```python
from build123d import *

# Parameters (mm, degrees)
SKETCH_1_W          = 56.4
SKETCH_1_H          = 20
EXTRUDE_1_DEPTH     = 8
SKETCH_2_R          = 2.25
CUT_EXTRUDE_1_DEPTH = 8
CHAMFER_1_SIZE      = 3
SKETCH_3_R          = 20
CUT_EXTRUDE_2_DEPTH = 8
SKETCH_4_W          = 5
SKETCH_4_H          = 8
CUT_EXTRUDE_3_DEPTH = 8


with BuildPart() as part:
    # 스케치1 → 보스-돌출1 (new body)
    with BuildSketch(Plane(origin=(0, 0, 0), x_dir=(1, 0, 0), z_dir=(0, 1, 0))):
        with Locations((28.2, 10)):
            Rectangle(SKETCH_1_W, SKETCH_1_H)
    extrude(amount=EXTRUDE_1_DEPTH)

    # 스케치2 → 컷-돌출1 (cut)
    with BuildSketch(Plane(origin=(0, 8, 0), x_dir=(1, 0, 0), z_dir=(0, 1, 0))):
        with Locations(Location((51.75, 15.35, 0), (0, 0, 270))):
            Circle(SKETCH_2_R)
        with Locations(Location((4.65, 15.35, 0), (0, 0, 270))):
            Circle(SKETCH_2_R)
    extrude(amount=-CUT_EXTRUDE_1_DEPTH, mode=Mode.SUBTRACT)

    # 모따기1
    chamfer_1_edges = [part.edges().sort_by_distance(p)[0] for p in [
        (56.4, 4, 0),
        (0, 4, 0),
    ]]
    chamfer(chamfer_1_edges, length=CHAMFER_1_SIZE)

    # 스케치3 → 컷-돌출2 (cut)
    with BuildSketch(Plane(origin=(0, 8, 0), x_dir=(1, 0, 0), z_dir=(0, 1, 0))):
        with Locations((28.2, -8.2)):
            Circle(SKETCH_3_R)
    extrude(amount=-CUT_EXTRUDE_2_DEPTH, mode=Mode.SUBTRACT)

    # 스케치4 → 컷-돌출3 (cut)
    with BuildSketch(Plane(origin=(0, 8, 0), x_dir=(1, 0, 0), z_dir=(0, 1, 0))):
        with Locations((13.2, 16)):
            Rectangle(SKETCH_4_W, SKETCH_4_H)
        with Locations((43.2, 16)):
            Rectangle(SKETCH_4_W, SKETCH_4_H)
    extrude(amount=-CUT_EXTRUDE_3_DEPTH, mode=Mode.SUBTRACT)


solid = part.part
```
Model file for the job. Use its own axes, mm. A direction names the side the tool comes from. Coordinates: 2 decimals unless noted, no trailing zeros. Loops run counter-clockwise (first coordinate to the right, second up) from the corner with the lowest first, then second, coordinate; pieces in that order, holes last. Notation, with made-up numbers: M -5.75,-35.5 L 49.25,-35.5 A11 cw 49.25,-19.5 Z; hole C -2.75,61.5 d6. An arc over 180 degrees is marked long. Use CSV: the item, a comma, the result in double quotes. Start each with the question number.
1. Band-saw the part on D-D, the plane z = -4.5. List the corners of the cut face in (x, y).
2. Two-plate mould, pull along X, no slides. Class faces 3 (the flat face through (0, 4, -11)), 4 (the cylindrical face through (53.98, 4.06, -15.64)), 5 (the flat face through (15.7, 4, -16)), 6 (the flat face through (54.9, 3.9, -1.5)): pulls with the +X half, pulls with the -X half, needs draft (parallel to the pull), parting line crosses it, or undercut.
3. Probe probe 1 along X at (y, z) = (4, -15.35); probe 2 along X at (y, z) = (5, -12.5); probe 3 along X at (y, z) = (7.75, -8.25). List the from-to ranges inside material, lowest first. Write a range as [from, to].
4. Band-saw the part on A-A, the plane x = 51.75. List the corners of the cut face in (y, z), then the cut area to 3 significant figures.
5. Tool access for faces 1 (the flat face through (40.7, 4, -16)), 2 (the flat face through (6, 4, 0)): list every direction of +Z, -Z, +X, -X, +Y, -Y with a clear straight run to the whole face (end or side of a thin tool).
6. Band-saw the part on C-C, the plane y = 4.25. List the corners of the cut face in (x, z), then the cut area to 3 significant figures.
7. Flat gauge pins, fed straight in: pin 1 (1.5 mm diameter, centred on x = 29, y = 5.5, fed in from +Z); pin 2 (2 mm diameter, centred on x = 24.5, y = 2, fed in from +Z); pin 3 (1.5 mm diameter, centred on x = 13.5, y = 5.5, fed in from -Z); pin 4 (4 mm diameter, centred on x = 4.65, z = -15.35, fed in from +Y). Where does each tip first touch, or does it go through?
8. Band-saw the part on B-B, the plane z = -14. List the corners of the cut face in (x, y).
Entries:
1,outline,"M 0,0 L 12.75,0 L 12.75,8 L 0,8 Z; M 43.65,0 L 56.4,0 L 56.4,8 L 43.65,8 Z"
2,face 3,"pulls with the -X half"
2,face 4,"undercut"
2,face 5,"undercut"
2,face 6,"pulls with the +X half"
3,probe 1,"x = [0, 2.4], [6.9, 10.7], [15.7, 40.7], [45.7, 49.5], [54, 56.4]"
3,probe 2,"x = [0, 10.7], [15.7, 40.7], [45.7, 56.4]"
3,probe 3,"x = [0, 16.82], [39.58, 56.4]"
4,outline,"M 0,-20 L 8,-20 L 8,-17.6 L 0,-17.6 Z; M 0,-13.1 L 8,-13.1 L 8,0 L 0,0 Z"
4,area,"124 mm2"
5,face 1,"-Z, +Y, -Y"
5,face 2,"+Z, +X, -X, +Y, -Y"
6,outline,"M 0,-20 L 10.7,-20 L 10.7,-12 L 15.7,-12 L 15.7,-20 L 40.7,-20 L 40.7,-12 L 45.7,-12 L 45.7,-20 L 56.4,-20 L 56.4,-3 L 53.4,0 L 46.44,0 A20 cw 9.96,0 L 3,0 L 0,-3 Z; hole C 4.65,-15.35 d4.5; hole C 51.75,-15.35 d4.5"
6,area,"697 mm2"
7,pin 1,"stops at z = -11.74"
7,pin 2,"stops at z = -11.24"
7,pin 3,"stops at z = -12"
7,pin 4,"passes through"
8,outline,"M 0,0 L 2.85,0 L 2.85,8 L 0,8 Z; M 6.45,0 L 10.7,0 L 10.7,8 L 6.45,8 Z; M 15.7,0 L 40.7,0 L 40.7,8 L 15.7,8 Z; M 45.7,0 L 49.95,0 L 49.95,8 L 45.7,8 Z; M 53.55,0 L 56.4,0 L 56.4,8 L 53.55,8 Z"
